from build123d import *

# Parameters (mm, degrees)
SKETCH7_W               = 86
SKETCH7_H               = 4
CUT_EXTRUDE3_DEPTH      = 122.688125961
CUT_EXTRUDE3_DEPTH_BACK = 122.688125961
SKETCH9_R               = 40
CUT_EXTRUDE4_DEPTH      = 122.688125961
SKETCH10_R              = 40
BOSS_EXTRUDE1_DEPTH     = 20
CUT_EXTRUDE7_DEPTH      = 124.255831505


with BuildPart() as part:
    # Sketch7 → Revolve4 (revolve)
    with BuildSketch(Plane.XY):
        with Locations((-43, -2)):
            Rectangle(SKETCH7_W, SKETCH7_H)
    revolve(axis=Axis((0, 0, 0), (0, -1, 0)))

    # Sketch9 → Cut-Extrude3 (cut, two sides: drawn at the far end of the back side and taken through both)
    with BuildSketch(Plane(origin=(0, 0, 0), x_dir=(1, 0, 0), z_dir=(0, 1, 0)).offset(-CUT_EXTRUDE3_DEPTH_BACK)):
        with Locations(Location((0, 0, 0), (0, 0, 270))):
            Circle(SKETCH9_R)
    extrude(amount=CUT_EXTRUDE3_DEPTH + CUT_EXTRUDE3_DEPTH_BACK, mode=Mode.SUBTRACT)

    # Sketch1 → Cut-Extrude4 (cut, through all)
    with BuildSketch(Plane(origin=(0, 0, 0), x_dir=(1, 0, 0), z_dir=(0, 1, 0))):
        with BuildLine():
            Line((-86.191983256, -25.902548569), (-9.566772234, -1.00550828))
            Line((-9.566772234, -1.00550828), (-89.693924294, 7.416194762))
            ThreePointArc((-89.693924294, 7.416194762), (-89.506970583, -9.407561694), (-86.191983256, -25.902548569))
        make_face()
    extrude(amount=-CUT_EXTRUDE4_DEPTH, mode=Mode.SUBTRACT)

    # Sketch10 → Boss-Extrude1 (add)
    with BuildSketch(Plane(origin=(0, 0, 0), x_dir=(-1, 0, 0), z_dir=(0, -1, 0))):
        with Locations(Location((0, 0, 0), (0, 0, 3.134016017))):
            Circle(SKETCH10_R)
    extrude(amount=BOSS_EXTRUDE1_DEPTH)

    # Sketch14 → Cut-Extrude7 (cut, through all)
    with BuildSketch(Plane(origin=(0, 0, 0), x_dir=(1, 0, 0), z_dir=(0, 1, 0))):
        Polygon((18.244865358, 22.530532352), (-22.530532352, 18.244865358), (-18.244865358, -22.530532352), (22.530532352, -18.244865358), align=None)
    extrude(amount=-CUT_EXTRUDE7_DEPTH, mode=Mode.SUBTRACT)


solid = part.part
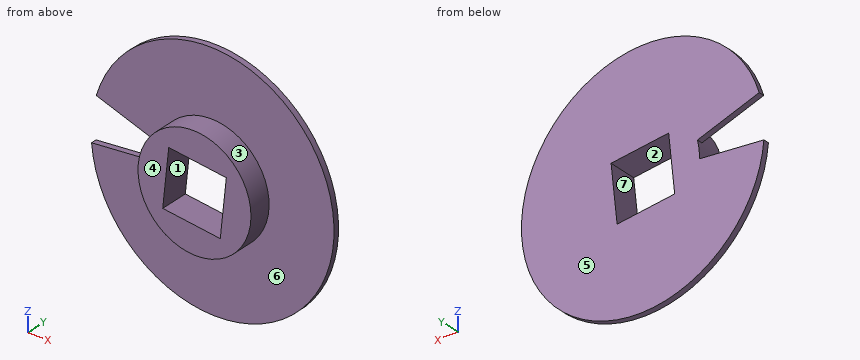
CAD build for the part. Positions are in the model's coordinates, mm. Face numbers are marked on the shaded views. A direction names the side the tool comes from. Round coordinates to 2 decimals unless told otherwise and drop trailing zeros. Write each loop counter-clockwise with the first axis right and the second up, starting at its lowest first coordinate (ties: lowest second). Pieces come first, ordered by that corner, then holes. Notation, with made-up numbers: M 32.25,84.5 L 40.25,84.5 A23 ccw 40.25,98.5 Z; hole C 33.5,-24 d8. An arc over 180 degrees is marked long. Use a Markdown table: item, result. Add a question column.
1. Slice it at B-B on z = 0. Give the cut face in (x, y), then the cut area to 3 significant figures.
2. Slice it at A-A on x = -53.5. Give the cut face in (y, z).
3. Drill centre lines: probe 1 along Y at (x, z) = (71.5, -1.5); probe 2 along X at (y, z) = (-6, 10.5); probe 3 along X at (y, z) = (-7.5, 14.5). Where is each one in solid material? Low to high.
4. Pull direction X, two halves, no side cores. Call the marked faces 1, 2, 3 and 4: released by +X, released by -X, zero draft, split by the parting line, or undercut.
5. 3-axis set-ups, long thin cutter, end or side, ignore diameter. For the marked faces 5, 6 and 7: which of +Z, -Z, +X, -X, +Y, -Y reach the whole face in a straight line?
6. Flat gauge pins, fed straight in: P1, Ø1.5, axis at y = -9.5, z = 21.5, coming from the +X side; P2, Ø1, axis at x = -63, z = -42, coming from the -Y side; P3, Ø12, axis at x = -10, y = -5.5, coming from the +Z side; P4, Ø3, axis at x = 51, z = 30, coming from the +Y side. Where does each tip first touch, or does it go through?
7. Slice it at C-C on y = -6. Give the cut face in (x, z).
8. Slice it at D-D on x = -28. Give the cut face in (y, z).
Reply:
| question | item | result |
|---|---|---|
| 1 | outline | M -40,-20 L -20.61,-20 L -20.61,0 L -40,0 Z; M 20.61,-20 L 40,-20 L 40,-4 L 86,-4 L 86,0 L 20.61,0 Z |
| 1 | area | 959 mm^2 |
| 2 | outline | M -4,-67.33 L 0,-67.33 L 0,-3.61 L -4,-3.61 Z; M -4,15.28 L 0,15.28 L 0,67.33 L -4,67.33 Z |
| 3 | probe 1 | y = -4 to 0 |
| 3 | probe 2 | x = -38.6 to -19.51, 21.72 to 38.6 |
| 3 | probe 3 | x = -37.28 to -19.09, 22.14 to 37.28 |
| 4 | face 1 | undercut |
| 4 | face 2 | undercut |
| 4 | face 3 | split by the parting line |
| 4 | face 4 | zero draft |
| 5 | face 5 | +Z, -Z, +X, -X, +Y |
| 5 | face 6 | -Y |
| 5 | face 7 | +Y, -Y |
| 6 | P1 | stops at x = 34.2 |
| 6 | P2 | stops at y = -4 |
| 6 | P3 | stops at z = 85.9 |
| 6 | P4 | stops at y = 0 |
| 7 | outline | C 0,0 d80; hole M -22.53,-18.24 L 18.24,-22.53 L 22.53,18.24 L -18.24,22.53 Z |
| 8 | outline | M -20,-28.57 L -4,-28.57 L -4,-81.31 L 0,-81.31 L 0,81.31 L -4,81.31 L -4,28.57 L -20,28.57 Z |
